Part model, mm, in its own coordinate system. Face numbers are marked on the shaded views. A direction names the side the tool comes from. Coordinates: 2 decimals unless noted, no trailing zeros. Loops run counter-clockwise (first coordinate to the right, second up) from the corner with the lowest first, then second, coordinate; pieces in that order, holes last. Notation, with made-up numbers: (-9.5, 59.5) - (35.5, 59.5) arc R17 ccw to (35.5, 81.5) - close; hole circle Ø5 at (3.5, 49.25). An arc over 180 degrees is marked (long way). Use a Markdown table: item, result. Add a question column.
1. Drop flat-ended pins along their axis: pin 1 (2 mm diameter, centred on y = 13, z = 18, fed in from +X); pin 2 (5 mm diameter, centred on x = 6, z = 25, fed in from -Y); pin 3 (3 mm diameter, centred on y = 14.68, z = 165.6, fed in from -X); pin 4 (4.5 mm diameter, centred on x = 9, z = 142, fed in from +Y). Give the stop position or say it passes through.
2. Wall check: probe 1 along Z at (x, y) = (9, 0.6); probe 2 along X at (y, z) = (0.55, 10); probe 3 along X at (y, z) = (0.55, 142). Give the ranges that are in metal, low to high. Write a range as [from, to].
3. Band-saw the part on B-B, the plane y = 14.68. Give the cut face in (x, z), plus the area to 3 significant figures.
4. Band-saw the part on C-C, the plane z = 42. Give the cut face in (x, y), plus the area to 3 significant figures.
5. Band-saw the part on D-D, the plane z = 147.5. Give the cut face in (x, y).
6. Band-saw the part on A-A, the plane x = 15.5. Give the cut face in (y, z), plus the area to 3 significant figures.
7. 3-axis set-ups, long thin cutter, end or side, ignore diameter. For the marked faces 1 and 2: which of +Z, -Z, +X, -X, +Y, -Y reach the whole face in a straight line?
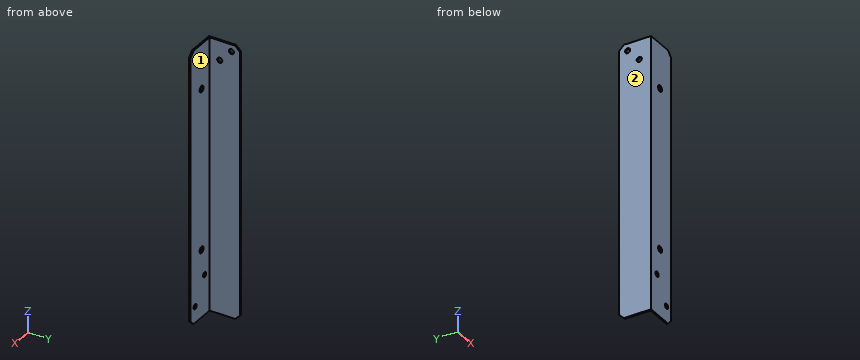
from build123d import *

# Parameters (mm, degrees)
BASE_DEPTH                      = 170
CHAMFEREDGES_SIZE               = 3
F_4_0_4_CABLE_TIE_HOLES_D       = 4
F_3_1_3_1_CABLECHAINSIDEHOLES_D = 3.2
F_3_2_3_2_CARRIAGESIDE_D        = 3.2


with BuildPart() as part:
    # Sketch1 → Base (new body)
    with BuildSketch(Plane.XY):
        Polygon((0, 0), (20, 0), (20, 1), (1, 1), (1, 20), (0, 20), align=None)
    extrude(amount=BASE_DEPTH)

    # ChamferEdges
    chamferedges_edges = [part.edges().sort_by_distance(p)[0] for p in [
        (20, 0.5, 170),
        (0.5, 20, 170),
        (0.5, 20, 0),
        (20, 0.5, 0),
    ]]
    chamfer(chamferedges_edges, length=CHAMFEREDGES_SIZE)

    # Ø4.0 (4) Cable tie Holes (through all)
    with Locations(Plane(origin=(0, 1, 0), x_dir=(1, 0, 0), z_dir=(0, 1, 0))):
        with Locations((9, -42), (9, -142)):
            Hole(F_4_0_4_CABLE_TIE_HOLES_D / 2)

    # Ø3.1 (3.1) CableChainSideHoles (through all)
    with Locations(Plane(origin=(1, 0, 0), x_dir=(0, 0, -1), z_dir=(1, 0, 0))):
        with Locations((-165.6, 14.68), (-157.8, 7.38)):
            Hole(F_3_1_3_1_CABLECHAINSIDEHOLES_D / 2)

    # Ø3.2 (3.2) CarriageSide (through all)
    with Locations(Plane(origin=(0, 1, 0), x_dir=(1, 0, 0), z_dir=(0, 1, 0))):
        with Locations((15.5, -10), (6, -25)):
            Hole(F_3_2_3_2_CARRIAGESIDE_D / 2)


solid = part.part
Geometry check:
| question | item | result |
|---|---|---|
| 1 | pin 1 | stops at x = 1 |
| 1 | pin 2 | stops at y = 0 |
| 1 | pin 3 | passes through |
| 1 | pin 4 | stops at y = 1 |
| 2 | probe 1 | z = [0, 40], [44, 140], [144, 170] |
| 2 | probe 2 | x = [0, 13.9], [17.1, 20] |
| 2 | probe 3 | x = [0, 7], [11, 20] |
| 3 | outline | (0, 0) - (1, 0) - (1, 164) - (0, 164) - close; (0, 167.2) - (1, 167.2) - (1, 170) - (0, 170) - close |
| 3 | area | 167 mm^2 |
| 4 | outline | (0, 0) - (7, 0) - (7, 1) - (1, 1) - (1, 20) - (0, 20) - close; (11, 0) - (20, 0) - (20, 1) - (11, 1) - close |
| 4 | area | 35.0 mm^2 |
| 5 | outline | (0, 0) - (20, 0) - (20, 1) - (1, 1) - (1, 20) - (0, 20) - close |
| 6 | outline | (0, 0) - (1, 0) - (1, 8.4) - (0, 8.4) - close; (0, 11.6) - (1, 11.6) - (1, 170) - (0, 170) - close |
| 6 | area | 167 mm^2 |
| 7 | face 1 | +Z, -Z, +X, +Y |
| 7 | face 2 | +Z, -Z, -X, +Y, -Y |
